The listing builds one solid part. Answer for the finished solid, in the listing's coordinates (mm). A direction names the side the tool comes from. Give positions to 0.01 mm unless a question says otherwise; leave off trailing zeros. Write each question's results on one line, items separated by ' | '. Start each with the question number.
Autodesk Inventor part; units mm, degrees
ref_plane "РабПлоскость1" through (-34.9651, 34.6315, 13) normal (0, 0, 1) x (1, 0, 0)
ref_plane "YZ Plane" through (0, 0, 0) normal (1, 0, 0) x (0, 1, 0)
ref_plane "XZ Plane" through (0, 0, 0) normal (0, 1, 0) x (-1, 0, 0)
sketch "Эскиз1" plane through (0, 0, 0) normal (0, 0, 1) x (1, 0, 0)
  circle A0 centre (-27.3933, 9.5988) radius 21.25
  circle A1 centre (-27.3933, 9.5988) radius 18.75
  point P0 (0, 0)
ref_plane "РабПлоскость1" through (-34.9651, 34.6315, 13) normal (0, 0, 1) x (1, 0, 0)
extrude "Выдавливание1" add sketch "Эскиз1" along normal up to surface (13 mm away) contours A0 | A1
ref_plane "РабПлоскость3" through (-27.3933, 9.5988, 13) normal (-1, 0, 0) x (0, -1, 0)
sketch "Эскиз3" plane through (-27.3933, 9.5988, 13) normal (-1, 0, 0) x (0, -1, 0)
  line L0 (-22.45, -4.27) -> (-21.25, -5.47)
  line L1 (-22.45, -3.07) -> (-22.45, -4.27)
  line L2 (30, -3.07) -> (-30, -3.07)
  line L3 (30, -3.07) -> (-30, -3.07)
  line L4 (-21.25, 0) -> (21.25, 0)
  line L5 (-21.25, 0) -> (-30, 0)
  line L6 (-30, 0) -> (-30, -3.07)
  line L7 (-30, -3.07) -> (-21.25, -3.07)
  line L8 (-21.25, -3.07) -> (-21.25, 0)
  line L9 (0, 0) -> (0, -13)
  line L10 (21.25, -13) -> (-21.25, -13)
  line L11 (-21.25, -13) -> (-21.25, 0)
  line L12 (0, 0) -> (-30, 0)
  line L13 (-30, 0) -> (-30, 11)
  line L14 (-30, 11) -> (0, 11)
  line L15 (0, 11) -> (0, 0)
  line L16 (-25.52, 6.93) -> (-25.52, -23)
  line L17 (-25.32, 6.93) -> (-25.32, -23)
  line L18 (-25.32, 6.93) -> (-25.32, 11)
  line L19 (-25.32, 6.93) -> (-30, 6.93)
  line L20 (-25.32, 7.23) -> (-30, 7.23)
  point P0 (9.5988, -13)
  point P1 (-21.25, -3.07)
  point P2 (-25.32, -3.07)
  dimension "d21" = 11
  dimension "d25" = 0.2
  dimension "d26" = 0.3
revolve "Вращение1" add sketch "Эскиз3" angle 360 about axis through (-27.3933, 9.5988, 13) along (0, 0, -1) contours L1 L2 L11 L0 | L2 L17 L5 L8 | L5 L17 L18 L14 L15 L4 | L20 L13 L14 L18
sketch "Эскиз5" plane through (-27.3933, 9.5988, 24) normal (0, 0, 1) x (1, 0, 0)
  circle A0 centre (0, 0) radius 22.45
  line L0 (-30.0943, 4.3007) -> (-34.526, 5.7406)
  arc A1 (-34.526, 5.7406) -> (-24.5579, -24.9382) centre (0, 0) ccw
  line L1 (-24.5579, -24.9382) -> (-21.8189, -21.1683)
  arc A2 (-21.8189, -21.1683) -> (-13.3898, -27.2924) centre (0, 0) ccw
  line L2 (-13.3898, -27.2924) -> (-16.1288, -31.0622)
  arc A3 (-16.1288, -31.0622) -> (16.1288, -31.0622) centre (0, 0) ccw
  line L3 (16.1288, -31.0622) -> (13.3898, -27.2924)
  arc A4 (13.3898, -27.2924) -> (21.8189, -21.1683) centre (0, 0) ccw
  line L4 (21.8189, -21.1683) -> (24.5579, -24.9382)
  arc A5 (24.5579, -24.9382) -> (34.526, 5.7406) centre (0, 0) ccw
  line L5 (34.526, 5.7406) -> (30.0943, 4.3007)
  arc A6 (30.0943, 4.3007) -> (26.8746, 14.2096) centre (0, 0) ccw
  line L6 (26.8746, 14.2096) -> (31.3064, 15.6496)
  arc A7 (31.3064, 15.6496) -> (5.2094, 34.6101) centre (0, 0) ccw
  line L7 (5.2094, 34.6101) -> (5.2094, 29.9503)
  arc A8 (5.2094, 29.9503) -> (-5.2094, 29.9503) centre (0, 0) ccw
  line L8 (-5.2094, 29.9503) -> (-5.2094, 34.6101)
  arc A9 (-5.2094, 34.6101) -> (-31.3064, 15.6496) centre (0, 0) ccw
  line L9 (-31.3064, 15.6496) -> (-26.8746, 14.2096)
  arc A10 (-26.8746, 14.2096) -> (-30.0943, 4.3007) centre (0, 0) ccw
  line L10 (3.8059, -20.9064) -> (6.2685, -34.4341)
  line L11 (18.7071, -10.0801) -> (30.8117, -16.6024)
  line L12 (21.0593, -2.8408) -> (34.6858, -4.679)
  line L13 (15.3675, 14.6766) -> (25.3112, 24.1732)
  line L14 (9.2094, 19.1507) -> (15.1685, 31.5423)
  line L15 (-9.2094, 19.1507) -> (-15.1685, 31.5423)
  line L16 (-15.3675, 14.6766) -> (-25.3112, 24.1732)
  line L17 (-21.0593, -2.8408) -> (-34.6858, -4.679)
  line L18 (-18.7071, -10.0801) -> (-30.8117, -16.6024)
  line L19 (-3.8059, -20.9064) -> (-6.2685, -34.4341)
  circle A11 centre (0, 0) radius 21.25
  line L20 (-9.2094, 19.1507) -> (-9.0121, 18.7403)
  line L21 (9.0121, 18.7403) -> (9.2094, 19.1507)
  line L22 (15.3675, 14.6766) -> (15.0382, 14.3621)
  line L23 (21.0593, -2.8408) -> (20.608, -2.7799)
  line L24 (18.7071, -10.0801) -> (18.3062, -9.864)
  line L25 (3.8059, -20.9064) -> (3.7243, -20.4584)
  line L26 (-3.8059, -20.9064) -> (-3.7243, -20.4584)
  line L27 (-18.7071, -10.0801) -> (-18.3062, -9.864)
  line L28 (-21.0593, -2.8408) -> (-20.608, -2.7799)
  line L29 (-15.3675, 14.6766) -> (-15.0382, 14.3621)
  arc A12 (-20.608, -2.7799) -> (-15.0382, 14.3621) centre (-21.9448, 7.1303) ccw
  arc A13 (-9.0121, 18.7403) -> (9.0121, 18.7403) centre (0, 23.0741) ccw
  arc A14 (15.0382, 14.3621) -> (20.608, -2.7799) centre (21.9448, 7.1303) ccw
  arc A15 (18.3062, -9.864) -> (3.7243, -20.4584) centre (13.5626, -18.6674) ccw
  arc A16 (-3.7243, -20.4584) -> (-18.3062, -9.864) centre (-13.5626, -18.6674) ccw
  point P0 (27.3933, -9.5988)
  dimension "d22" = 10
extrude "Выдавливание3" cut sketch "Эскиз5" against normal up to surface (14.07 mm away) contours A0 L12 A11 L13 | A0 L13 A7 L6 A6 L5 A5 L12 | L14 A11 L15 A0 | A0 L15 A9 L8 A8 L7 A7 L14 | A11 L23 A14 L22 | L11 A5 L4 A4 L3 A3 L10 A0 | A0 L10 A11 L11 | L21 A13 L20 A11 | A11 L25 A15 L24 | L16 A11 L17 A0 | A0 L17 A1 L0 A10 L9 A9 L16 | L19 A3 L2 A2 L1 A1 L18 A0 | A0 L18 A11 L19 | L29 A12 L28 A11 | A11 L27 A16 L26
sketch "Эскиз6" plane through (-27.3933, 9.5988, 13) normal (-1, 0, 0) x (0, -1, 0)
  line L0 (16.6287, -10.8787) -> (-16.6287, -10.8787)
  line L1 (-21.25, -13) -> (21.25, -13)
  line L2 (-18.75, -13) -> (-16.6287, -10.8787)
  line L3 (18.75, -13) -> (16.6287, -10.8787)
  line L4 (21.25, -13) -> (-21.25, -13)
  line L5 (-21.25, -13) -> (-19.25, -13)
  line L6 (-19.25, -13) -> (-17.1287, -10.8787)
  line L7 (0, -10.8787) -> (0, -10.3787)
  line L8 (0, -10.3787) -> (-16.6287, -10.3787)
  line L9 (-16.6287, -10.3787) -> (-17.1287, -10.8787)
  line L10 (0, -10.3787) -> (0, -13)
  line L11 (0, -13) -> (-19.25, -13)
  line L12 (-19.25, -13) -> (-19.25, -10.1)
  line L13 (-19.25, -10.1) -> (0, -10.1)
  line L14 (0, -10.3787) -> (0, -10.1)
  point P0 (20.25, -13)
  point P1 (-19.25, -13)
  dimension "d29" = 2
  dimension "d30" = 135
  dimension "d31" = 0.5
  dimension "d44" = 2.9
revolve "Вращение2" cut sketch "Эскиз6" angle 360 about axis through (-27.3933, 9.5988, 2.6213) along (0, 0, -1) contours L10 L1 L2 L0 | L0 L2 L1 L6 L9 L8 L7 | L8 L9 L6 L12 L13 L14
sketch "Эскиз7" plane through (-27.3933, 32.6729, 24) normal (0, 0, 1) x (1, 0, 0)
  circle A0 centre (0, -23.0741) radius 22.45
  circle A1 centre (0, -23.0741) radius 1.6
  line L0 (0, -23.0741) -> (0, -31.0741)
  circle A2 centre (0, -31.0741) radius 1.6
  circle A3 centre (7.6085, -25.5463) radius 1.6
  circle A4 centre (4.7023, -16.602) radius 1.6
  circle A5 centre (-4.7023, -16.602) radius 1.6
  circle A6 centre (-7.6085, -25.5463) radius 1.6
  point P0 (27.3933, -32.6729)
  dimension "d33" = 3.2
  dimension "d34" = 8
  dimension "d37" = 360
extrude "Выдавливание4" cut sketch "Эскиз7" against normal blind 30 contours A1 | A2 | A3 | A4 | A5 | A6
chamfer "Фаска1" distance 2 angle 45 6 edges at (-28.9933, 1.5988, 24) (-36.6017, 7.1266, 24) (-33.6955, 16.0709, 24) (-28.9933, 9.5988, 24) (-24.291, 16.0709, 24) (-21.3848, 7.1266, 24)
properties part number "tire cap"
1. Each of these flat-tipped pins is pushed along its axis until it touches: pin 1 Ø1.5 at (x, z) = (-21, 2.5) entering from -Y; pin 2 Ø5 at (x, y) = (-12, 33) entering from -Z; pin 3 Ø2 at (y, z) = (-7.5, 11) entering from +X. Where does it stop, or does it pass through?
2. Consider probe 1 along X at (y, z) = (17, 8.5); probe 2 along Z at (x, y) = (-13, 0); probe 3 along Z at (x, y) = (-9, 7). Determine where each line is inside the solid, lowest interval first. Write a range as [from, to].
3. The mould has two halves that part along Y. Classify faces 1 (the flat face through (-44, 32, 20.23)), 2 (the cylindrical face through (-15.006, 13.789, 17.063)), 3 (the cylindrical face through (1.115, 0.256, 22.141)): pulls with the +Y half, pulls with the -Y half, needs draft (parallel to the pull), parting line crosses it, or undercut.
4. A tool of negligible diameter and unlimited length cuts with its end or side. For faces 4 (the flat face through (-11, 32, 20.23)), 5 (the cylindrical face through (-27.33, -15.72, 15.01)), 6 (the flat face through (-28, 27, 9.93)), from which of +Z, -Z, +X, -X, +Y, -Y can it reach the whole face along a straight path? Write none if from no direction.
5. Section A-A (z = 18.75) is taken. Give the number of separate pieces and of enclosed holes in the cut face, then the cut area to 3 significant figures.
Results:
1) pin 1: stops at y = -10.89 | pin 2: stops at z = 20.23 | pin 3: stops at x = -23.5
2) probe 1: x = [-48.34, -33.4], [-30.79, -23.99], [-21.39, -6.44] | probe 2: z = [2.9, 9.93] | probe 3: z = [2.9, 24]
3) face 1: needs draft | face 2: undercut | face 3: pulls with the -Y half
4) face 4: -Z, +X, +Y | face 5: -Z, -Y | face 6: +Z, +Y
5) separate pieces: 1 | enclosed holes: 6 | area: 1,010 mm²
